Can you work these out from the drawing? Everything is in mm from the part's minimum corner. Give positions to 0.01 mm unless a question says otherwise; leave off trailing zeros. Write each loop counter-clockwise with the first axis right and the second up, starting at its lowest first coordinate (ties: lowest second). Pieces come first, ordered by that corner, then holes. Notation, with made-up numbers: (-39.5, 12) -> (-9.5, 12) arc R19 ccw to (-9.5, 16) -> close; hole circle Ø6 at (12, -27). An arc over 180 degrees is marked (long way). Use one line per item in the form item = value.
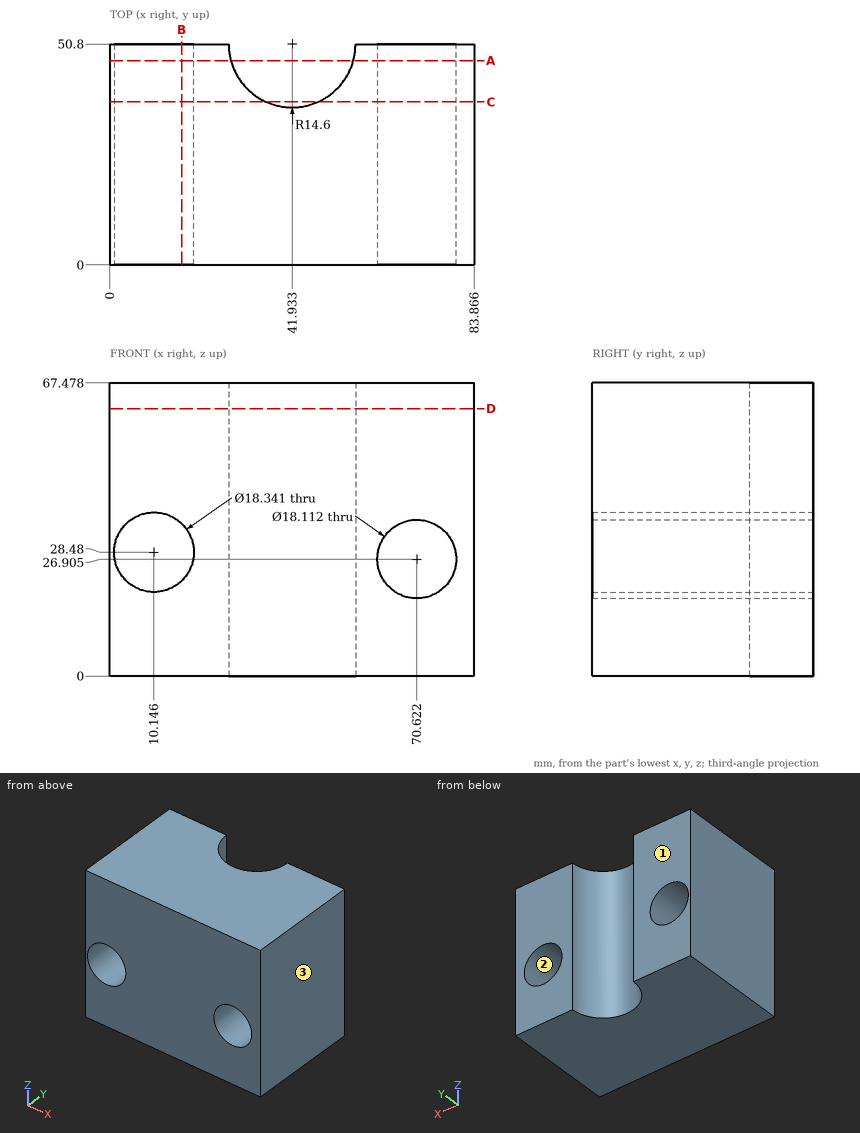
Q1. If we mould it in two halves opening along X, with no side actions, what happens to the marked faces 1, 2 and 3? For each: +X half, -X half, draft (parallel to the pull), parting line (faces both ways), or undercut.
Result set:
face_1 = draft
face_2 = undercut
face_3 = +X half
Q2. I want a section at D-D, the plane z = 61.5. Write out the boundary of the cut face in (x, y).
Result set:
outline = (0, 0) -> (83.87, 0) -> (83.87, 50.8) -> (56.53, 50.8) arc R14.6 cw to (27.33, 50.8) -> (0, 50.8) -> close
Q3. I want a section at C-C, the plane y = 37.5. Write out the boundary of the cut face in (x, z) (1 decimal).
Result set:
outline = (0, 0) -> (35.9, 0) -> (35.9, 67.5) -> (0, 67.5) -> close; (48, 0) -> (83.9, 0) -> (83.9, 67.5) -> (48, 67.5) -> close; hole circle Ø18.3 at (10.1, 28.5); hole circle Ø18.1 at (70.6, 26.9)
Q4. If I drill on line 1 along X through (y, z) = (12, 25) (1 decimal); line 2 along Z through (x, y) = (7.5, 21); line 3 along Z through (x, y) = (66, 23.5), over which ranges is the centre line in solid material (lowest first)? Write a range as from..to.
Result set:
line_1 = 0..1.7, 18.6..61.8, 79.5..83.9
line_2 = 0..19.7, 37.26..67.48
line_3 = 0..19.12, 34.69..67.48
Q5. I want a section at B-B, the plane x = 16.5. Write out the boundary of the cut face in (y, z), and give its area (3 significant figures).
Result set:
outline = (0, 0) -> (50.8, 0) -> (50.8, 21.87) -> (0, 21.87) -> close; (0, 35.09) -> (50.8, 35.09) -> (50.8, 67.48) -> (0, 67.48) -> close
area = 2,760 mm2
Q6. I want a section at A-A, the plane y = 47. Write out the boundary of the cut face in (x, z) (1 decimal).
Result set:
outline = (0, 0) -> (27.8, 0) -> (27.8, 67.5) -> (0, 67.5) -> close; (56, 0) -> (83.9, 0) -> (83.9, 67.5) -> (56, 67.5) -> close; hole circle Ø18.3 at (10.1, 28.5); hole circle Ø18.1 at (70.6, 26.9)
Q7. Will this pin go through, and if not, where does the flat tip stop? pin 1 Ø6 at (x, z) = (49, 14) entering from +Y (1 decimal).
Result set:
pin_1 = 40.2
